Here's how the part is built. I have some questions about the finished solid (model axes, mm). Face numbers are marked on the shaded views. Give positions to 0.01 mm unless a question says otherwise; leave off trailing zeros. Write each loop counter-clockwise with the first axis right and the second up, starting at its lowest first coordinate (ties: lowest second). Pieces come first, ordered by that corner, then holes. Notation, with made-up numbers: (14.5, 45) -> (37.5, 45) arc R32 ccw to (37.5, 80) -> close; hole circle Ø5 at (70.25, 28.25). An arc over 180 degrees is marked (long way). Use one line per item in the form item = value.
```python
from build123d import *

# Parameters (mm, degrees)
SKETCH1_W           = 178
SKETCH1_H           = 118
SKETCH1_W_2         = 159.5
SKETCH1_H_2         = 99.5
BOSS_EXTRUDE1_DEPTH = 4
SKETCH2_W           = 178
SKETCH2_H           = 118
SKETCH2_W_2         = 170
SKETCH2_H_2         = 110
BOSS_EXTRUDE2_DEPTH = 15
FILLET1_R           = 3


with BuildPart() as part:
    # Sketch1 → Boss-Extrude1 (new body)
    with BuildSketch(Plane(origin=(0, 0, 0), x_dir=(1, 0, 0), z_dir=(0, 1, 0))):
        with Locations((2.365202132, 0)):
            Rectangle(SKETCH1_W, SKETCH1_H)
        Rectangle(SKETCH1_W_2, SKETCH1_H_2, mode=Mode.SUBTRACT)
    extrude(amount=BOSS_EXTRUDE1_DEPTH)

    # Sketch2 → Boss-Extrude2 (add)
    with BuildSketch(Plane.XZ):
        with Locations((2.365202132, 0)):
            Rectangle(SKETCH2_W, SKETCH2_H)
        with Locations((2.365202132, 0)):
            Rectangle(SKETCH2_W_2, SKETCH2_H_2, mode=Mode.SUBTRACT)
    extrude(amount=BOSS_EXTRUDE2_DEPTH)

    # Fillet1
    fillet1_edges = [part.edges().sort_by_distance(p)[0] for p in [
        (-86.634797868, -5.5, -59),
        (91.365202132, -5.5, -59),
        (91.365202132, -5.5, 59),
        (-86.634797868, -5.5, 59),
    ]]
    fillet(fillet1_edges, radius=FILLET1_R)


solid = part.part
```
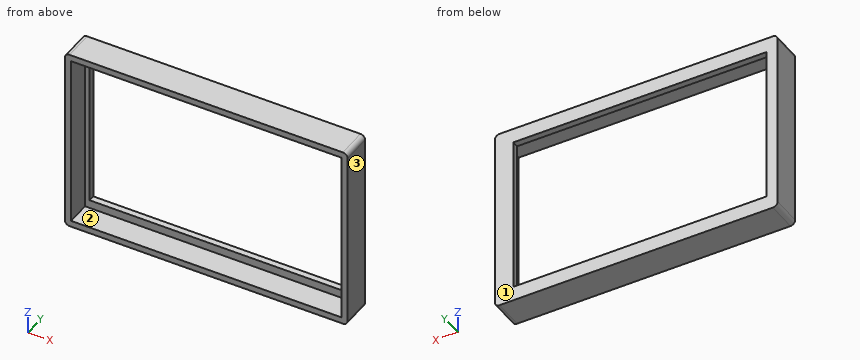
Q1. If I drill on line 1 along Z through (x, y) = (50, -10.25); line 2 along X through (y, z) = (-8, 19); line 3 along Z through (x, y) = (50.5, 2.5), over which ranges is the centre line in solid material (lowest first)? Write a range as from..to.
Result set:
line_1 = -59..-55, 55..59
line_2 = -86.63..-82.63, 87.37..91.37
line_3 = -59..-49.75, 49.75..59
Q2. I want a section at B-B, the plane y = -2. Write out the boundary of the cut face in (x, z), and give its area (3 significant figures).
Result set:
outline = (-86.63, -56) arc R3 ccw to (-83.63, -59) -> (88.37, -59) arc R3 ccw to (91.37, -56) -> (91.37, 56) arc R3 ccw to (88.37, 59) -> (-83.63, 59) arc R3 ccw to (-86.63, 56) -> close; hole (-82.63, -55) -> (87.37, -55) -> (87.37, 55) -> (-82.63, 55) -> close
area = 2,300 mm2
Q3. I want a section at A-A, the plane z = 2.5. Write out the boundary of the cut face in (x, y), and give its area (3 significant figures).
Result set:
outline = (-86.63, -15) -> (-82.63, -15) -> (-82.63, 0) -> (-79.75, 0) -> (-79.75, 4) -> (-86.63, 4) -> close; (79.75, 0) -> (87.37, 0) -> (87.37, -15) -> (91.37, -15) -> (91.37, 4) -> (79.75, 4) -> close
area = 194 mm2
Q4. I want a section at C-C, the plane x = 35. Write out the boundary of the cut face in (y, z).
Result set:
outline = (-15, -59) -> (4, -59) -> (4, -49.75) -> (0, -49.75) -> (0, -55) -> (-15, -55) -> close; (-15, 55) -> (0, 55) -> (0, 49.75) -> (4, 49.75) -> (4, 59) -> (-15, 59) -> close
Q5. If we mould it in two halves opening along X, with no side actions, what happens to the marked faces 1, 2 and 3? For each: +X half, -X half, draft (parallel to the pull), parting line (faces both ways), or undercut.
Result set:
face_1 = draft
face_2 = undercut
face_3 = +X half
